Input: part model. Units: mm. Frame: model coordinates. Round coordinates to 2 decimals unless told otherwise and drop trailing zeros. Loops run counter-clockwise (first coordinate to the right, second up) from the corner with the lowest first, then second, coordinate; pieces in that order, holes last. Notation, with made-up numbers: (85.25, 43) -> (108.25, 43) arc R17 cw to (108.25, 71) -> close; hole circle Ø11 at (6.25, -14.5). An arc over 180 degrees is marked (long way). Answer in a Markdown table with one row per item. Add a question column.
Q1. Section A-A, the plane z = 118. Output: boundary loops of the cut face in (x, y).
Q2. Pin query (flat end, axial travel): pin 1 (3 mm diameter, centred on x = 0, y = 0, fed in from +Z); pin 2 (8 mm diameter, centred on y = 5, z = 7, fed in from +X); pin 3 (4 mm diameter, centred on x = -4.5, z = 73, fed in from +Y); pin 4 (2 mm diameter, centred on x = 5, z = -183.5, fed in from -Y). Return the tip coordinate at first contact, or that it passes through.
Q3. Ray query, L1, parallel to Y at x = 0, z = -314.25; L2, parallel to X at y = 0, z = -314.25; L3, parallel to Y at x = -4, z = 26. Return the intervals inside material, ascending. Write a range as from..to.
Autodesk Inventor part; units mm, degrees
ref_plane "YZ Plane" through (0, 0, 0) normal (1, 0, 0) x (0, 1, 0)
ref_plane "XZ Plane" through (0, 0, 0) normal (0, 1, 0) x (-1, 0, 0)
ref_plane "XY Plane" through (0, 0, 0) normal (0, 0, 1) x (1, 0, 0)
sketch "Sketch1" plane through (0, 0, 0) normal (0, 0, 1) x (1, 0, 0)
  line L0 (0, 7.3323) -> (6.35, 3.6662)
  line L1 (6.35, 3.6662) -> (6.35, -3.6662)
  line L2 (6.35, -3.6662) -> (0, -7.3323)
  line L3 (0, -7.3323) -> (-6.35, -3.6662)
  line L4 (-6.35, -3.6662) -> (-6.35, 3.6662)
  line L5 (-6.35, 3.6662) -> (0, 7.3323)
  point P0 (0, 0)
  point P1 (0, 0)
  dimension "d1" = 12.7
extrude "Extrusion1" add sketch "Sketch1" along normal mid plane 638.048
sketch "Sketch2" plane through (0, 0, 319.024) normal (0, 0, 1) x (1, 0, 0)
  point P0 (0, 0)
hole "Hole1" at (0, 0, 319.024) direction (0, 0, -1) diameter 4.9784 depth 19.05 tip angle 118
mirror "Mirror1" about plane through (0, 0, 0) normal (0, 0, 1) of "Hole1"
properties part number "0.5_Bottom_INTAKE_SHAFT" material "Aluminum, 6061-T6"
Answer block:
| question | item | result |
|---|---|---|
| 1 | outline | (-6.35, -3.67) -> (0, -7.33) -> (6.35, -3.67) -> (6.35, 3.67) -> (0, 7.33) -> (-6.35, 3.67) -> close |
| 2 | pin 1 | z = 299.38 |
| 2 | pin 2 | x = 6.35 |
| 2 | pin 3 | y = 5.89 |
| 2 | pin 4 | y = -5.02 |
| 3 | L1 | -7.33..-2.49, 2.49..7.33 |
| 3 | L2 | -6.35..-2.49, 2.49..6.35 |
| 3 | L3 | -5.02..5.02 |
